The model under review builds one solid part; all positions refer to its coordinate system, in mm. A direction names the side the tool comes from. Round coordinates to 2 decimals unless told otherwise and drop trailing zeros. Loops run counter-clockwise (first coordinate to the right, second up) from the corner with the lowest first, then second, coordinate; pieces in that order, holes last. Notation, with made-up numbers: M 56,-9.5 L 69,-9.5 A17 ccw 69,-2.5 Z; hole C 88,-32.5 d10. An arc over 180 degrees is marked long. Answer in a Markdown table with one row per item. Add a question column.
Autodesk Inventor part; units mm, degrees
ref_plane "YZ Plane" through (0, 0, 0) normal (1, 0, 0) x (0, 1, 0)
ref_plane "XZ Plane" through (0, 0, 0) normal (0, 1, 0) x (-1, 0, 0)
ref_plane "XY Plane" through (0, 0, 0) normal (0, 0, 1) x (1, 0, 0)
sketch "Sketch1" plane through (0, 0, 0) normal (0, 1, 0) x (-1, 0, 0)
  point P0 (0, 0)
sketch "Sketch2" plane through (0, 0, 0) normal (0, 1, 0) x (-1, 0, 0)
  point P0 (0, 0)
sketch "Sketch3" plane through (0, 0, 0) normal (0, 1, 0) x (-1, 0, 0)
  circle A0 centre (0, 0) radius 2.54
  dimension "d0" = 5.08
extrude "Extrusion1" add sketch "Sketch3" along normal blind 25.4
thread "Thread1"
sketch "Sketch4" plane through (0, 25.4, 0) normal (0, 1, 0) x (1, 0, 0)
  circle A0 centre (0, 0) radius 3.175
  dimension "d5" = 6.35
extrude "Extrusion2" add sketch "Sketch4" along normal blind 1.524
fillet "Fillet1" radius 3.175 1 edges at (-3.175, 26.924, 0)
properties part number "1inchscrew"
1. For pin 1 Ø1 at (y, z) = (14.5, -2) entering from -X; pin 2 Ø1.9 at (x, z) = (0.5, -1.5) entering from -Y; pin 3 Ø3 at (x, z) = (-2.5, 0.5) entering from +Y, all flat-tipped, find the tip position at first contact; note any pin that passes through.
2. Machinability: for faces 1 (the cylindrical face through (0.33, 12.52, -2.52)), 2 (the flat face through (0, 0, 0)), which of the approach directions +Z, -Z, +X, -X, +Y, -Y give a long, thin tool a straight path to every point of the face, cutting with its end or side? Answer none if there is none.
3. To check wall thickness, follow probe 1 along Z at (x, y) = (0, 23.75); probe 2 along Z at (x, y) = (1, 19.5); probe 3 along Y at (x, z) = (0.5, 1.5). State the ranges of each line that lie inside material, in increasing order.
4. Take a section at A-A, the plane y = 24.5. State the section outline as (x, z) points, and give its area (3 significant figures).
Check sheet entries:
| question | item | result |
|---|---|---|
| 1 | pin 1 | stops at x = -2.05 |
| 1 | pin 2 | stops at y = 0 |
| 1 | pin 3 | stops at y = 26.87 |
| 2 | face 1 | -Y |
| 2 | face 2 | +Z, -Z, +X, -X, -Y |
| 3 | probe 1 | z = -2.54 to 2.54 |
| 3 | probe 2 | z = -2.33 to 2.33 |
| 3 | probe 3 | y = 0 to 26.72 |
| 4 | outline | C 0,0 d5.08 |
| 4 | area | 20.3 mm^2 |
